The listing builds one solid part. Answer for the finished solid, in the listing's coordinates (mm). A direction names the side the tool comes from. Coordinates: 2 decimals unless noted, no trailing zeros. Order: outer loops, then holes, each group sorted by start corner. A loop starts at its lowest first (then second) coordinate and runs counter-clockwise, first axis right, second up.
```python
from build123d import *

# Parameters (mm, degrees)
SALIENTE_EXTRUIR2_DEPTH = 4
SALIENTE_EXTRUIR3_DEPTH = 4
REDONDEO1_R             = 10
REDONDEO2_R             = 10
CROQUIS4_R              = 1.6
CORTAR_EXTRUIR1_DEPTH   = 21.5


with BuildPart() as part:
    # Croquis2 → Saliente-Extruir2 (new, symmetric)
    with BuildSketch(Plane.XY):
        with BuildLine():
            ThreePointArc((3.679760923, -1.486719918), (-0.5866186, -3.925156708), (-3.953647708, -0.345899354))
            Line((-3.953647708, -0.345899354), (-6.229010011, 25.661610777))
            Line((-6.229010011, 25.661610777), (-6.229010011, 55.661610777))
            Line((-6.229010011, 55.661610777), (-14.085344509, 55.661610777))
            Line((-14.085344509, 55.661610777), (-14.085344509, 25.661610777))
            Line((-14.085344509, 25.661610777), (-6.96875, 0))
            ThreePointArc((-6.96875, 0), (-1.329700187, -6.840714435), (6.461312487, -2.610539698))
            ThreePointArc((6.461312487, -2.610539698), (5.632446595, -0.657854026), (3.679760923, -1.486719918))
        make_face()
    extrude(amount=SALIENTE_EXTRUIR2_DEPTH, both=True)

    # Croquis3 → Saliente-Extruir3 (add, symmetric)
    with BuildSketch(Plane.XY):
        Polygon((-10.527047254, 12.830805389), (-6.757235143, -1.70389254), (-3.584372578, -1.70389254), (-6.327047254, 12.830805389), align=None)
    extrude(amount=SALIENTE_EXTRUIR3_DEPTH, both=True)

    # Redondeo1
    redondeo1_edges = [part.edges().sort_by_distance(p)[0] for p in [
        (-14.085344509, 25.661610777, 0),
    ]]
    fillet(redondeo1_edges, radius=REDONDEO1_R)

    # Redondeo2
    # the kernel refuses this fillet: 10 mm, written as the material it adds along each edge
    with BuildSketch(Plane(origin=(-6.229010011, 25.661610777, -4), x_dir=(0, 1, 0), z_dir=(0, 0, 1))) as redondeo2_piece_1:
        with BuildLine():
            CenterArc((REDONDEO2_R * 0.0436609429085, -REDONDEO2_R), REDONDEO2_R, 90, 5)
            Line((-REDONDEO2_R * 0.0434947998391, -REDONDEO2_R * 0.00380530190825), (0, 0))
            Line((0, 0), (REDONDEO2_R * 0.0436609429085, 0))
        make_face()
    extrude(amount=8)

    # Croquis4 → Cortar-Extruir1 (cut)
    with BuildSketch(Plane.ZY.offset(14.085344509)):
        with Locations(Location((-0.25, 48.661610777, 0), (0, 0, 270))):
            Circle(CROQUIS4_R)
    extrude(amount=-CORTAR_EXTRUIR1_DEPTH, mode=Mode.SUBTRACT)


solid = part.part
```
1) For faces 1 (the flat face through (-3.815, -0.484, 0.056)), 2 (the flat face through (-6.229, 41, 0)), 3 (the flat face through (-12.147, 18.671, 0.056)), determine the directions among +Z, -Z, +X, -X, +Y, -Y from which every point of the face is accessible in a straight line to the end or side of a thin tool.
2) A cutting plane is placed at D-D, the plane x = 2.5. Write down the section's boundary in (y, z), plus the area to 3 significant figures.
3) A cutting plane is placed at B-B, the plane y = 30. Write down the section's boundary in (x, z).
4) Straight lines are drawn through the part: probe 1 along X at (y, z) = (52.5, 0.75); probe 2 along Y at (x, z) = (-0.25, 0.25); probe 3 along X at (y, z) = (9.5, 1). For each, find the intervals that lie inside material, in ascending order.
5) Each of these flat-tipped pins is pushed along its axis until it touches: P1, Ø2, axis at x = 2, z = 2.5, coming from the +Y side; P2, Ø1.5, axis at x = 1.5, z = 3, coming from the -Y side. Where does it stop, or does it pass through?
6) A cutting plane is placed at A-A, the plane z = -0.25. Write down the section's boundary in (x, y), plus the area to 3 significant figures.
7) The mould has two halves that part along Y. Classify faces 4 (the flat face through (-14.085, 42, 0)), 5 (the cylindrical face through (-13.991, 25.655, 0.056)), 6 (the cylindrical face through (-10.21, 49.84, 0.83)): released by +Y, released by -Y, zero draft, split by the parting line, or undercut.
8) A cutting plane is placed at C-C, the plane x = -9.75. Write down the section's boundary in (y, z).
Working result:
1. face 1: +Z, -Z, +Y
1. face 2: +Z, -Z, +X, +Y
1. face 3: +Z, -Z, -X, -Y
2. outline: (-6.5, -4) - (-3.08, -4) - (-3.08, 4) - (-6.5, 4) - close
2. area: 27.4 mm2
3. outline: (-14.09, -4) - (-6.23, -4) - (-6.23, 4) - (-14.09, 4) - close
4. probe 1: x = -14.09 to -6.23
4. probe 2: y = -6.96 to -3.96
4. probe 3: x = -9.66 to -4.82
5. P1: stops at y = -2.6
5. P2: stops at y = -6.93
6. outline: (-14.09, 27.02) arc R10 ccw to (-13.72, 24.35) - (-10.53, 12.83) - (-6.76, -1.7) arc R6.97 ccw to (6.46, -2.61) arc R1.5 ccw to (3.68, -1.49) arc R3.97 cw to (-3.58, -1.7) - (-4.05, 0.77) - (-6.19, 25.23) arc R10 cw to (-6.23, 26.1) - (-6.23, 47.06) - (-14.09, 47.06) - close; (-14.09, 50.26) - (-6.23, 50.26) - (-6.23, 55.66) - (-14.09, 55.66) - close
6. area: 400 mm2
7. face 4: zero draft
7. face 5: released by -Y
7. face 6: undercut
8. outline: (9.83, -4) - (55.66, -4) - (55.66, 4) - (9.83, 4) - close; hole circle Ø3.2 at (48.66, -0.25)
